Read the model definition and answer for the solid it produces. Units are mm, in the model's axes. A direction names the side the tool comes from. Coordinates: 2 decimals unless noted, no trailing zeros. Write each loop counter-clockwise with the first axis right and the second up, starting at its lowest first coordinate (ties: lowest second). Pieces come first, ordered by that corner, then holes. Notation, with made-up numbers: (-34, -28) -> (-15, -28) arc R29 ccw to (-15, 8) -> close; hole circle Ø3 at (44, 43.5). An arc over 180 degrees is marked (long way). Return JSON: item names as keys, results as strings.
from build123d import *

# Parameters (mm, degrees)
SKETCH3_W           = 50
SKETCH3_H           = 50
SKETCH3_W_2         = 44
SKETCH3_H_2         = 44
BOSS_EXTRUDE1_DEPTH = 1052.5
SKETCH4_W           = 40
SKETCH4_H           = 2
BOSS_EXTRUDE2_DEPTH = 40
SKETCH5_R           = 5
CUT_EXTRUDE1_DEPTH  = 1000
FILLET1_R           = 20


with BuildPart() as part:
    # Sketch3 → Boss-Extrude1 (new, symmetric)
    with BuildSketch(Plane.XY):
        Rectangle(SKETCH3_W, SKETCH3_H)
        Rectangle(SKETCH3_W_2, SKETCH3_H_2, mode=Mode.SUBTRACT)
    extrude(amount=BOSS_EXTRUDE1_DEPTH, both=True)

    # Sketch4 → Boss-Extrude2 (add)
    with BuildSketch(Plane(origin=(0, 25, 0), x_dir=(1, 0, 0), z_dir=(0, 1, 0))):
        with Locations((0, 448.5)):
            Rectangle(SKETCH4_W, SKETCH4_H)
        with Locations((0, 426.5)):
            Rectangle(SKETCH4_W, SKETCH4_H)
        with Locations((0, -461.5)):
            Rectangle(SKETCH4_W, SKETCH4_H)
        with Locations((0, -483.5)):
            Rectangle(SKETCH4_W, SKETCH4_H)
    extrude(amount=BOSS_EXTRUDE2_DEPTH)

    # Sketch5 → Cut-Extrude1 (cut)
    with BuildSketch(Plane.XY.offset(484.5)):
        with Locations((0, 45)):
            Circle(SKETCH5_R)
    extrude(amount=-CUT_EXTRUDE1_DEPTH, mode=Mode.SUBTRACT)

    # Fillet1
    fillet1_edges = [part.edges().sort_by_distance(p)[0] for p in [
        (-20, 65, -448.5),
        (-20, 65, -426.5),
        (-20, 65, 461.5),
        (-20, 65, 483.5),
    ]]
    fillet(fillet1_edges, radius=FILLET1_R)


solid = part.part
1. Flat-ended cylindrical pins translate along their axes: pin 1 Ø1 at (y, z) = (45, -449) entering from +X; pin 2 Ø12 at (x, y) = (-9.5, 54.5) entering from -Z; pin 3 Ø0.6 at (y, z) = (38, 483.5) entering from -X. Find the tip coordinate at first contact, or state that the pin passes through.
Taken from the geometry:
{"pin 1": "stops at x = 20", "pin 2": "stops at z = -449.5", "pin 3": "stops at x = -20"}
2. A tool of negligible diameter and unlimited length cuts with its end or side. For faces 1 (the face through (-22.3, 0.1, -1052.5)), 2 (the face through (4, 40, 460.5)), 3 (the face through (4, 40, 484.5)), 4 (the face through (4, 40, -449.5)), 5 (the face through (0, -22, 15)), from which of +Z, -Z, +X, -X, +Y, -Y can it reach the whole face along a straight path? Write none if from no direction.
Taken from the geometry:
{"face 1": "-Z, +X, -X, +Y, -Y", "face 2": "+X, -X, +Y", "face 3": "+Z, +X, -X, +Y", "face 4": "-Z, +X, -X, +Y", "face 5": "+Z, -Z"}
3. For a pull along Y with two mould halves and no side action, classify faces 6 (the face through (0, 25, 15)), 7 (the face through (0, 22, 15)), 8 (the face through (-22.3, 0.1, 1052.5)), 9 (the face through (0, -25, 15)) as +Y half, -Y half, draft (parallel to the pull), parting line (faces both ways), or undercut.
Taken from the geometry:
{"face 6": "+Y half", "face 7": "undercut", "face 8": "draft", "face 9": "-Y half"}
4. The part is cut by section A-A (z = 656.5). Determine the outline of the cut face in (x, y), then the cut area to 3 significant figures.
Taken from the geometry:
{"outline": "(-25, -25) -> (25, -25) -> (25, 25) -> (-25, 25) -> close; hole (-22, -22) -> (22, -22) -> (22, 22) -> (-22, 22) -> close", "area": "564 mm2"}
5. Consider L1, parallel to Y at x = 0, z = 483.9; L2, parallel to Z at x = -13.5, y = 37; L3, parallel to Y at x = 2.5, z = 26. Determine where each line is inside the solid, lowest interval first.
Taken from the geometry:
{"L1": "y = -25 to -22, 22 to 40, 50 to 65", "L2": "z = -449.5 to -447.5, -427.5 to -425.5, 460.5 to 462.5, 482.5 to 484.5", "L3": "y = -25 to -22, 22 to 25"}
